```python
from build123d import *

# Parameters (mm, degrees)
SKETCH_2_R      = 1.5
SKETCH_2_R_2    = 10
EXTRUDE_2_DEPTH = 3


with BuildPart() as part:
    # 草图2 → 凸台-拉伸2 (new body)
    with BuildSketch(Plane.XY):
        with BuildLine():
            Line((-72.904615241, 0), (73, 0))
            ThreePointArc((73, 0), (77.949747468, 2.050252532), (80, 7))
            Line((80, 7), (80, 60))
            Line((80, 60), (105, 60))
            ThreePointArc((105, 60), (110.7284389, 62.976942983), (111.584524662, 69.375717782))
            Line((111.584524662, 69.375717782), (76.970149392, 165.31270549))
            ThreePointArc((76.970149392, 165.31270549), (74.373778179, 168.711112108), (70.295901401, 170))
            Line((70.295901401, 170), (-70.295901401, 170))
            ThreePointArc((-70.295901401, 170), (-74.373778179, 168.711112108), (-76.970149392, 165.31270549))
            Line((-76.970149392, 165.31270549), (-111.584524662, 69.375717782))
            ThreePointArc((-111.584524662, 69.375717782), (-110.7284389, 62.976942983), (-105, 60))
            Line((-105, 60), (-80, 60))
            Line((-80, 60), (-80, 7.095384759))
            ThreePointArc((-80, 7.095384759), (-77.921809919, 2.078190081), (-72.904615241, 0))
        make_face()
        with Locations((-30.952307621, 7.065749953)):
            Circle(SKETCH_2_R, mode=Mode.SUBTRACT)
        with Locations(Location((31.047692379, 7.065749953, 0), (0, 0, 180))):
            Circle(SKETCH_2_R, mode=Mode.SUBTRACT)
        with Locations((-25.452307621, 64.065749953)):
            Circle(SKETCH_2_R, mode=Mode.SUBTRACT)
        with Locations(Location((25.547692379, 64.065749953, 0), (0, 0, 180))):
            Circle(SKETCH_2_R, mode=Mode.SUBTRACT)
        with Locations((-72.441382232, 165.375717782)):
            Circle(SKETCH_2_R, mode=Mode.SUBTRACT)
        with Locations((-106.29148568, 65.75613767)):
            Circle(SKETCH_2_R, mode=Mode.SUBTRACT)
        with Locations(Location((106.29148568, 65.75613767, 0), (0, 0, 180))):
            Circle(SKETCH_2_R, mode=Mode.SUBTRACT)
        with Locations(Location((72.441382232, 165.375717782, 0), (0, 0, 180))):
            Circle(SKETCH_2_R, mode=Mode.SUBTRACT)
        with Locations((-75, 3.552033702)):
            Circle(SKETCH_2_R, mode=Mode.SUBTRACT)
        with Locations(Location((75, 3.552033702, 0), (0, 0, 180))):
            Circle(SKETCH_2_R, mode=Mode.SUBTRACT)
        with Locations((80, 100)):
            Circle(SKETCH_2_R_2, mode=Mode.SUBTRACT)
    extrude(amount=EXTRUDE_2_DEPTH)


solid = part.part
```
Could you check a few things on this model? Use its own coordinates, in mm. Coordinates: 2 decimals unless noted, no trailing zeros. Order: outer loops, then holes, each group sorted by start corner. A loop starts at its lowest first (then second) coordinate and runs counter-clockwise, first axis right, second up. Notation, with made-up numbers: M 77,86.25 L 127,86.25 A23 ccw 127,97.25 Z; hole C 31,68 d11. An arc over 180 degrees is marked long. Use a Markdown table: item, result. Add a question column.
Q1. I want a section at D-D on y = 76. List the corners of the cut face in (x, z) for me.
Q2. We'd pull the mould along Y, two halves only. Please class faces 1 (the cylindrical face through (72.63, 106.76, 1.48)), 2 (the flat face through (-94.035, 118.016, 1.479)), 3 (the cylindrical face through (-110.78, 63.05, 1.48)), 4 (the cylindrical face through (77.9, 2, 1.5)): pulls with the +Y half, pulls with the -Y half, needs draft (parallel to the pull), parting line crosses it, or undercut.
Q3. If I drill on L1, parallel to Y at x = 75, z = 2.25; L2, parallel to X at y = 31.5, z = 2; L3, parallel to X at y = 102.5, z = 0.45, over which ranges is the centre line in solid material (lowest first)?
Q4. I want a section at B-B on z = 1.75. Give the number of separate pieces and of enclosed holes in the cut face, then the cut area to 3 significant figures.
Q5. I want a section at C-C on y = 148. List the corners of the cut face in (x, z) for me, then the cut area to 3 significant figures.
Q6. I want a section at A-A on y = 107. List the corners of the cut face in (x, z) for me.
Q7. I'm going to push flat-ended pins straight in: pin 1 (18 mm diameter, centred on x = 80, y = 100, fed in from +Z); pin 2 (5 mm diameter, centred on x = 25.55, y = 64.07, fed in from -Z); pin 3 (0.9 mm diameter, centred on x = -97, z = 2, fed in from -Y); pin 4 (1.5 mm diameter, centred on y = 28.5, z = 1.5, fed in from -X). Where does each tip first touch, or does it pass through?
Checked values:
| question | item | result |
|---|---|---|
| 1 | outline | M -109.19,0 L 109.19,0 L 109.19,3 L -109.19,3 Z |
| 2 | face 1 | undercut |
| 2 | face 2 | pulls with the +Y half |
| 2 | face 3 | parting line crosses it |
| 2 | face 4 | pulls with the -Y half |
| 3 | L1 | 0.29 to 2.05, 5.05 to 91.34, 108.66 to 168.22 |
| 3 | L2 | -80 to 80 |
| 3 | L3 | -99.63 to 70.32, 89.68 to 99.63 |
| 4 | separate pieces | 1 |
| 4 | enclosed holes | 11 |
| 4 | area | 30,100 mm² |
| 5 | outline | M -83.22,0 L 83.22,0 L 83.22,3 L -83.22,3 Z |
| 5 | area | 499 mm² |
| 6 | outline | M -98.01,0 L 72.86,0 L 72.86,3 L -98.01,3 Z; M 87.14,0 L 98.01,0 L 98.01,3 L 87.14,3 Z |
| 7 | pin 1 | through |
| 7 | pin 2 | z = 0 |
| 7 | pin 3 | y = 60 |
| 7 | pin 4 | x = -80 |
